Check sheet for the modelled part. Datum: model origin and axes. Units: mm. A direction names the side the tool comes from. Coordinates: 2 decimals unless noted, no trailing zeros. Loops run counter-clockwise (first coordinate to the right, second up) from the corner with the lowest first, then second, coordinate; pieces in that order, holes last.
```python
from build123d import *

# Parameters (mm, degrees)
EXTRUDE_1_DEPTH = 1.5
SKETCH_2_R      = 3
EXTRUDE_2_DEPTH = 7
EXTRUDE_START   = 3.5
EXTRUDE_3_DEPTH = 1.5
SKETCH_3_R      = 2.5
EXTRUDE_4_DEPTH = 23
SKETCH_4_R      = 2
EXTRUDE_5_DEPTH = 19.5
CHAMFER_1_SIZE  = 0.39


with BuildPart() as part:
    # Эскиз1 → Бобышка-Вытянуть1 (new body)
    with BuildSketch(Plane.XY):
        Polygon((-4, 2.309401077), (-4, -2.309401077), (0, -4.618802154), (4, -2.309401077), (4, 2.309401077), (0, 4.618802154), align=None)
    extrude(amount=EXTRUDE_1_DEPTH)

    # Эскиз2 → Бобышка-Вытянуть2 (add)
    with BuildSketch(Plane.XY.offset(1.5)):
        Circle(SKETCH_2_R)
    extrude(amount=EXTRUDE_2_DEPTH)

    # Эскиз1<2> → Бобышка-Вытянуть3 (add)
    with BuildSketch(Plane.XY.offset(EXTRUDE_START)):
        Polygon((-4, 2.309401077), (-4, -2.309401077), (0, -4.618802154), (4, -2.309401077), (4, 2.309401077), (0, 4.618802154), align=None)
    extrude(amount=EXTRUDE_3_DEPTH)

    # Эскиз3 → Бобышка-Вытянуть4 (add)
    with BuildSketch(Plane.XY.offset(8.5)):
        Circle(SKETCH_3_R)
    extrude(amount=EXTRUDE_4_DEPTH)

    # Эскиз4 → Бобышка-Вытянуть5 (add)
    with BuildSketch(Plane.XY.offset(31.5)):
        Circle(SKETCH_4_R)
    extrude(amount=EXTRUDE_5_DEPTH)

    # Фаска1
    chamfer_1_edges = [part.edges().sort_by_distance(p)[0] for p in [
        (-2, 0, 51),
    ]]
    chamfer(chamfer_1_edges, length=CHAMFER_1_SIZE)


solid = part.part
```
1) Mould release check, pull along Z, two halves, no side actions. Record for faces 3 (the flat face through (0, 0, 51)), 4 (the flat face through (-1.97, 3.48, 4.24)), 5 (the cylindrical face through (-3, 0, 2)): +Z half, -Z half, draft (parallel to the pull), parting line (faces both ways), or undercut.
Answer sheet:
face 3: +Z half
face 4: draft
face 5: undercut
2) Section check B-B on y = 0. Enter the section's corners in (x, z).
Answer sheet:
outline: (-4, 0) - (4, 0) - (4, 1.5) - (3, 1.5) - (3, 3.5) - (4, 3.5) - (4, 5) - (3, 5) - (3, 8.5) - (2.5, 8.5) - (2.5, 31.5) - (2, 31.5) - (2, 50.61) - (1.61, 51) - (-1.61, 51) - (-2, 50.61) - (-2, 31.5) - (-2.5, 31.5) - (-2.5, 8.5) - (-3, 8.5) - (-3, 5) - (-4, 5) - (-4, 3.5) - (-3, 3.5) - (-3, 1.5) - (-4, 1.5) - close
3) Depth check by flat-ended pin: pin 1 (5 mm diameter, centred on y = 0.5, z = 29, fed in from -X); pin 2 (1.5 mm diameter, centred on x = -2.5, y = -0.5, fed in from +Z); pin 3 (2 mm diameter, centred on x = 3, z = 16, fed in from +Y). Enter the tip coordinate at first touch or a pass-through.
Answer sheet:
pin 1: stops at x = -2.5
pin 2: stops at z = 50.81
pin 3: stops at y = 1.5
4) Set-up check for faces 1 (the flat face through (-2, 2, 8.5)), 2 (the flat face through (-1.97, 3.48, 0.74)): record each of +Z, -Z, +X, -X, +Y, -Y from which the full face is reachable in a straight line by a thin tool's end or side.
Answer sheet:
face 1: +Z
face 2: +Z, -Z, -X, +Y
5) Section check C-C on z = 10.5. Enter the section's corners in (x, y).
Answer sheet:
outline: circle Ø5 at (0, 0)
6) Section check A-A on y = 3.75. Enter the section's corners in (x, z), plus the area to 3 significant figures.
Answer sheet:
outline: (-1.5, 0) - (1.5, 0) - (1.5, 1.5) - (-1.5, 1.5) - close; (-1.5, 3.5) - (1.5, 3.5) - (1.5, 5) - (-1.5, 5) - close
area: 9.03 mm2
7) Scan lines: line 1 (Z direction, x = -0.5, y = -3.25); line 2 (Z direction, x = 2.5, y = 0.75); line 3 (Z direction, x = -2, y = -0.75). Record each from-to range of solid material in increasing order.
Answer sheet:
line 1: z = 0 to 1.5, 3.5 to 5
line 2: z = 0 to 8.5
line 3: z = 0 to 31.5
8) Section check D-D on y = -4. Enter the section's corners in (x, z), plus the area to 3 significant figures.
Answer sheet:
outline: (-1.07, 0) - (1.07, 0) - (1.07, 1.5) - (-1.07, 1.5) - close; (-1.07, 3.5) - (1.07, 3.5) - (1.07, 5) - (-1.07, 5) - close
area: 6.43 mm2
